Design review of the part built by this model. Coordinates are the model's own, in mm. A direction names the side the tool comes from. Coordinates: 2 decimals unless noted, no trailing zeros. Write each loop counter-clockwise with the first axis right and the second up, starting at its lowest first coordinate (ties: lowest second). Pieces come first, ordered by that corner, then holes. Notation, with made-up numbers: (44.5, -3.5) - (49.5, -3.5) arc R9 ccw to (49.5, 11.5) - close; hole circle Ø5 at (55.5, 77.5). An arc over 180 degrees is marked (long way). Use a Markdown table: item, result.
Solid Edge part; units mm, degrees
sketch "Sketch1" plane through (0, 0, 0) normal (0, 0, 1) x (1, 0, 0)
  line L0 (35, -80) -> (35, 80)
  line L1 (35, 80) -> (-35, 80)
  line L2 (-35, 80) -> (-35, -80)
  line L3 (-35, -80) -> (35, -80)
extrude "Protrusion1" add sketch "Sketch1" against normal blind 10
sketch "Sketch2" plane through (0, 0, 0) normal (0, 0, 1) x (1, 0, 0)
  line L0 (-24.8754, 70) -> (25.1246, 70)
  line L1 (25.1246, 70) -> (25.1246, -30)
  line L2 (25.1246, -30) -> (-24.8754, -30)
  line L3 (-24.8754, -30) -> (-24.8754, 70)
extrude "Recorte_Extrudado_1" cut sketch "Sketch2" against normal blind 5
sketch "Sketch3" plane through (0, 0, 0) normal (0, 0, 1) x (0, -1, 0)
  line L0 (40, 15.1246) -> (40, -14.8754)
  line L1 (40, -14.8754) -> (70, -14.8754)
  line L2 (70, -14.8754) -> (70, 15.1246)
  line L3 (70, 15.1246) -> (40, 15.1246)
extrude "Recorte_Extrudado_2" cut sketch "Sketch3" against normal blind 5
fillet "Redondo_1" radius 1 1 edges at (25.1246, -30, -2.5)
fillet "Redondo_2" radius 1 7 edges at (-24.8754, -30, -2.5) (25.1246, 70, -2.5) (-24.8754, 70, -2.5) (15.1246, -40, -2.5) (-14.8754, -40, -2.5) (15.1246, -70, -2.5) (-14.8754, -70, -2.5)
fillet "Redondo_3" radius 3 4 edges at (-35, -80, -5) (35, -80, -5) (35, 80, -5) (-35, 80, -5)
sketch "Sketch4" plane through (0, 0, 0) normal (0, 0, 1) x (1, 0, 0)
  line L0 (-4.8754, -80) -> (-4.8754, -70)
  line L1 (-4.8754, -70) -> (5.1246, -70)
  line L2 (5.1246, -70) -> (5.1246, -80)
  line L3 (5.1246, -80) -> (-4.8754, -80)
extrude "Recorte_Extrudado_3" cut sketch "Sketch4" against normal blind 5
fillet "Redondo_4" radius 0.5 4 edges at (5.1246, -70, -2.5) (-4.8754, -70, -2.5) (-4.8754, -80, -2.5) (5.1246, -80, -2.5)
(1) For pin 1 (8 mm diameter, centred on x = -1.5, y = 60, fed in from +Z); pin 2 (4 mm diameter, centred on x = 1, z = -1.5, fed in from -Y), all flat-tipped, find the tip position at first contact; note any pin that passes through.
Determined:
| item | result |
|---|---|
| pin 1 | z = -5 |
| pin 2 | y = -40 |
(2) Draft analysis for pull direction X (two halves, no side actions). For faces 1 (the cylindrical face through (-34.1, -79.14, -5.07)), 2 (the flat face through (15.125, -55, -2)), 3 (the flat face through (0, -34, 0)), state which applies: +X half, -X half, draft (parallel to the pull), parting line (faces both ways), or undercut.
Determined:
| item | result |
|---|---|
| face 1 | -X half |
| face 2 | undercut |
| face 3 | draft |
(3) Take a section at C-C on y = -18. Write out the cut boundary in (x, z), and give its area (3 significant figures).
Determined:
| item | result |
|---|---|
| outline | (-35, -10) - (35, -10) - (35, 0) - (25.12, 0) - (25.12, -5) - (-24.88, -5) - (-24.88, 0) - (-35, 0) - close |
| area | 450 mm2 |
(4) Machinability: for faces 4 (the flat face through (5.125, -75, -2)), 5 (the flat face through (-24.875, 19, -2)), 6 (the cylindrical face through (34.1, 79.14, -5.07)), which of the approach directions +Z, -Z, +X, -X, +Y, -Y give a long, thin tool a straight path to every point of the face, cutting with its end or side? Answer none if there is none.
Determined:
| item | result |
|---|---|
| face 4 | +Z, -Y |
| face 5 | +Z |
| face 6 | +Z, -Z, +X, +Y |
(5) Take a section at B-B on x = 21.5. Write out the cut boundary in (y, z), and give its area (3 significant figures).
Determined:
| item | result |
|---|---|
| outline | (-80, -10) - (80, -10) - (80, 0) - (70, 0) - (70, -5) - (-30, -5) - (-30, 0) - (-80, 0) - close |
| area | 1,100 mm2 |
(6) For L1, parallel to Y at x = 8, z = -1.5; L2, parallel to Y at x = 17.5, z = -3; L3, parallel to X at y = -44.5, z = -2.5, list the stretches that pass through material, from the lowest coordinate up. Write a range as from..to.
Determined:
| item | result |
|---|---|
| L1 | -80..-70, -40..-30, 70..80 |
| L2 | -80..-30, 70..80 |
| L3 | -35..-14.88, 15.12..35 |
